Geometry: see drawing. Coordinates: mm, zero at the bounding-box minimum. A direction names the side the tool comes from. Coordinates: 2 decimals unless noted, no trailing zeros. Order: outer loops, then holes, each group sorted by start corner. A loop starts at its lowest first (then second) coordinate and runs counter-clockwise, first axis right, second up. Notation, with made-up numbers: M -34,-31.5 L -20,-31.5 A31 cw -20,-5.5 Z; hole C 15,-6.5 d10. An arc over 180 degrees is marked long. Answer in a Markdown table with one row per item.
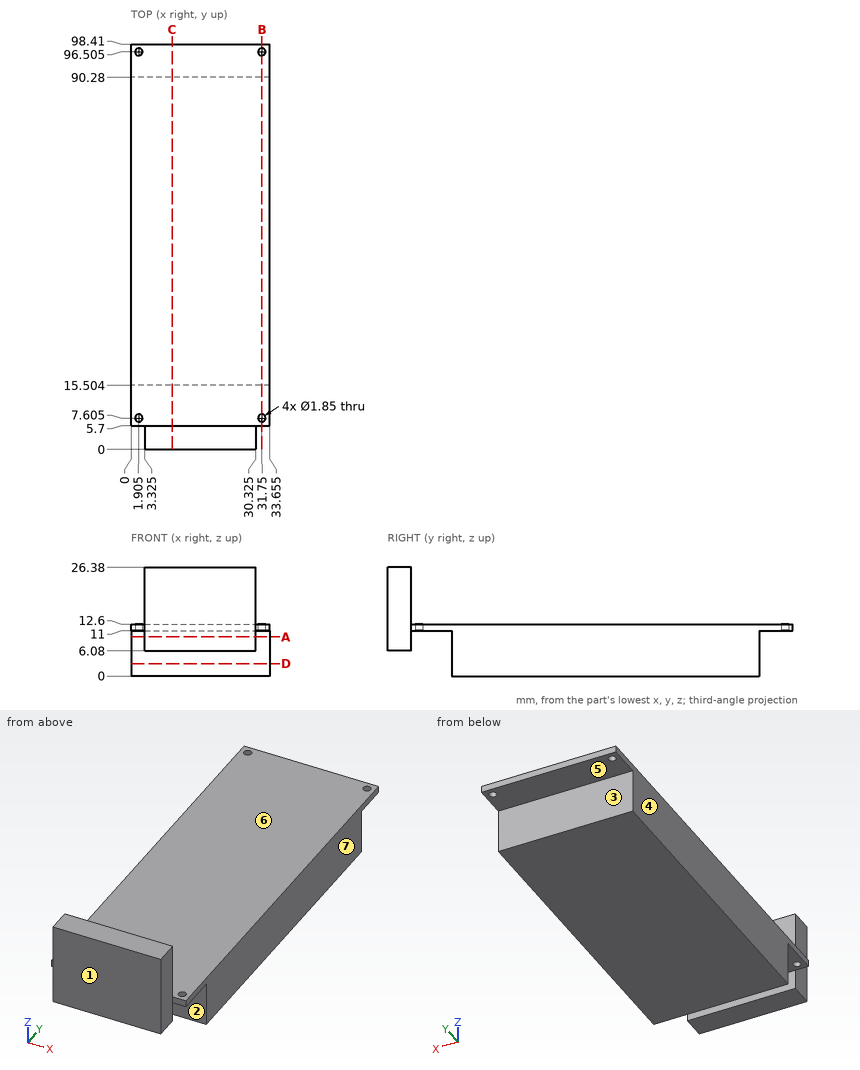
1) Contact query for flat-ended pins moving along their axis: pin 1 (3.5 mm diameter, centred on x = 11.5, z = 3.5, fed in from -Y); pin 2 (5 mm diameter, centred on x = 14, y = 10, fed in from -Z); pin 3 (1.3 mm diameter, centred on x = 31.5, z = 11.5, fed in from -Y); pin 4 (1.1 mm diameter, centred on x = 31.75, y = 96.505, fed in from +Z). Output: stop coordinate, or through.
Resolved:
| item | result |
|---|---|
| pin 1 | stops at y = 15.5 |
| pin 2 | stops at z = 11 |
| pin 3 | stops at y = 5.7 |
| pin 4 | passes through |
2) Cut plane D-D, the plane z = 3. Output: boundary loops of the cut face in (x, y) (1 decimal), and give its area (3 significant figures).
Resolved:
| item | result |
|---|---|
| outline | M 0,15.5 L 33.7,15.5 L 33.7,90.3 L 0,90.3 Z |
| area | 2,520 mm2 |
3) Material intervals for probe 1 along Y at (x, z) = (31.75, 12); probe 2 along Y at (x, z) = (12, 8.25) (1 decimal); probe 3 along Z at (x, y) = (12, 5), sorted ascending.
Resolved:
| item | result |
|---|---|
| probe 1 | y = 5.7 to 6.68, 8.53 to 95.58, 97.43 to 98.41 |
| probe 2 | y = 0 to 5.7, 15.5 to 90.3 |
| probe 3 | z = 6.08 to 26.38 |
4) Cut plane A-A, the plane z = 9.5. Output: boundary loops of the cut face in (x, y) (1 decimal), and give its area (3 significant figures).
Resolved:
| item | result |
|---|---|
| outline | M 0,15.5 L 33.7,15.5 L 33.7,90.3 L 0,90.3 Z; M 3.3,0 L 30.3,0 L 30.3,5.7 L 3.3,5.7 Z |
| area | 2,670 mm2 |
5) Cut plane C-C, the plane x = 10. Output: boundary loops of the cut face in (y, z) (1 decimal).
Resolved:
| item | result |
|---|---|
| outline | M 0,6.1 L 5.7,6.1 L 5.7,11 L 15.5,11 L 15.5,0 L 90.3,0 L 90.3,11 L 98.4,11 L 98.4,12.6 L 5.7,12.6 L 5.7,26.4 L 0,26.4 Z |
6) Reachability of the marked faces 5, 6 and 7 from +Z, -Z, +X, -X, +Y, -Y: full face, straight path, thin tool, end or side. Return the list, or none.
Resolved:
| item | result |
|---|---|
| face 5 | -Z, +X, -X, +Y |
| face 6 | +Z, +X, -X, +Y |
| face 7 | +Z, -Z, +X, +Y, -Y |
7) Cut plane B-B, the plane x = 31.75. Output: boundary loops of the cut face in (y, z) (1 decimal).
Resolved:
| item | result |
|---|---|
| outline | M 5.7,11 L 6.7,11 L 6.7,12.6 L 5.7,12.6 Z; M 8.5,11 L 15.5,11 L 15.5,0 L 90.3,0 L 90.3,11 L 95.6,11 L 95.6,12.6 L 8.5,12.6 Z; M 97.4,11 L 98.4,11 L 98.4,12.6 L 97.4,12.6 Z |
8) Mould query, pull axis Y, two halves, no side actions, for the marked faces 1, 2, 3 and 4. Classes: +Y half, -Y half, draft (parallel to the pull), parting line (faces both ways), or undercut.
Resolved:
| item | result |
|---|---|
| face 1 | -Y half |
| face 2 | undercut |
| face 3 | +Y half |
| face 4 | draft |
